Design review of the part shown in the three views and the two pictorial views. Dimensions are in mm from the part's minimum x, y and z. Give positions to 0.01 mm unless a question says otherwise; leave off trailing zeros. Order: outer loops, then holes, each group sorted by start corner. A loop starts at its lowest first (then second) coordinate and runs counter-clockwise, first axis right, second up.
Item 1: Consider section C-C (y = 6.35). Give the number of separate pieces and of enclosed holes in the cut face, plus the area to 3 significant figures.
Item 2: For P1, Ø6, axis at x = 10, y = 6.5, coming from the +Z side; P2, Ø3, axis at x = 5.5, y = 6, coming from the -Z side; P3, Ø1.5, axis at y = 7.5, z = 36, coming from the +X side; P4, Ø2, axis at y = 6.35, z = 6.8, coming from the -X side, all flat-tipped, find the tip position at first contact; note any pin that passes through.
Item 3: The part is to be moulded in two halves that separate along Y. For the marked faces 1, 2 and 3, say which applies: released by +Y, released by -Y, zero draft, split by the parting line, or undercut.
Item 4: Consider section A-A (z = 6.8). Give the boundary of the cut face in (x, y), plus the area to 3 significant figures.
Item 5: Consider section D-D (z = 44.4). Give the boundary of the cut face in (x, y).
Item 6: For probe 1 along Y at (x, z) = (6.35, 5.75); probe 2 along Z at (x, y) = (11.5, 5); probe 3 along Y at (x, z) = (7.25, 44.4), list the stretches that pass through material, from the lowest coordinate up.
Item 7: Consider section B-B (x = 1.25). Give the boundary of the cut face in (y, z).
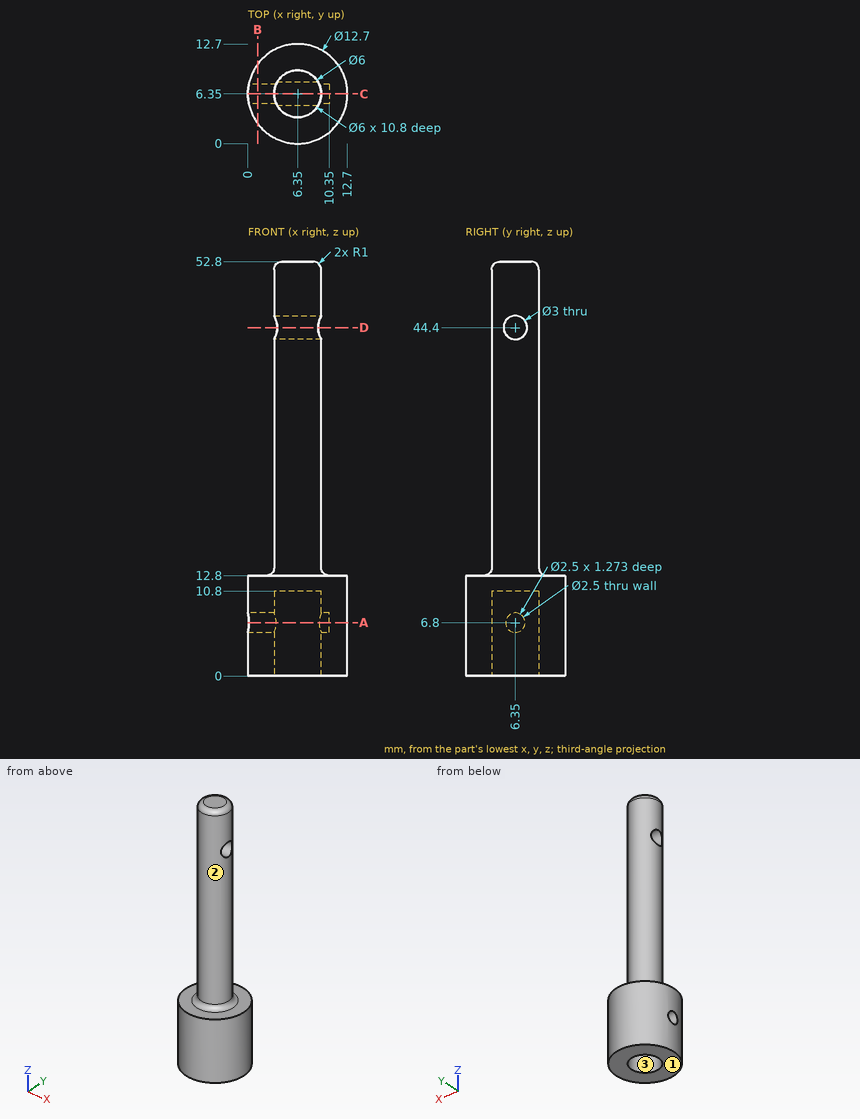
Resolved:
1. separate pieces: 3
1. enclosed holes: 0
1. area: 309 mm2
2. P1: stops at z = 52.8
2. P2: stops at z = 10.8
2. P3: stops at x = 9.32
2. P4: stops at x = 10.35
3. face 1: zero draft
3. face 2: split by the parting line
3. face 3: undercut
4. outline: (0.12, 5.1) arc R6.35 ccw (long way) to (0.12, 7.6) - (3.62, 7.6) arc R3 cw to (9.08, 7.6) - (10.35, 7.6) - (10.35, 5.1) - (9.08, 5.1) arc R3 cw to (3.62, 5.1) - close
4. area: 87.2 mm2
5. outline: (3.75, 4.85) arc R3 ccw to (8.95, 4.85) - close; (3.75, 7.85) - (8.95, 7.85) arc R3 ccw to start
6. probe 1: y = 0 to 3.35, 9.35 to 12.7
6. probe 2: z = 0 to 12.8
6. probe 3: y = 3.49 to 4.85, 7.85 to 9.21
7. outline: (2.57, 0) - (10.13, 0) - (10.13, 12.8) - (2.57, 12.8) - close; hole circle Ø2.5 at (6.35, 6.8)
